Work out the finished part from the listing and answer in its coordinate system (mm). Give positions to 0.01 mm unless a question says otherwise; leave off trailing zeros. Write each loop counter-clockwise with the first axis right and the second up, starting at its lowest first coordinate (ties: lowest second). Pieces come first, ordered by that corner, then holes.
1) Find section A-A (z = 2.5). Determine the outline of the cut face in (x, y), plus the area to 3 significant figures.
2) Determine the mould class of faces 1 (the face through (2.49, -0.13, 3.49)), 2 (the face through (2.5, 0, 4)), 3 (the face through (-38, 0, -3)) for opening direction Z: pulls with the +Z half, pulls with the -Z half, needs draft (parallel to the pull), parting line crosses it, or undercut.
3) Given pin 1 Ø4 at (x, z) = (-20.5, -3) entering from +Y; pin 2 Ø3 at (y, z) = (0, -7.5) entering from -X; pin 3 Ø3 at (x, y) = (-32, 0.5) entering from +Z, each flat-ended and moving along its own axis, determine where each tip first touches the part or whether it passes through.
4) Find section C-C (x = -18.5). Determine the outline of the cut face in (y, z), plus the area to 3 significant figures.
5) Find section B-B (y = -0.4). Determine the outline of the cut face in (x, z), plus the area to 3 significant figures.
6) Straight lines are drawn through the part: probe 1 along Z at (x, y) = (2.7, 0); probe 2 along Y at (x, z) = (2.45, -7.5); probe 3 along X at (y, z) = (-1.15, -1.75). For each, find the intervals that lie inside material, in ascending order.
7) Find section D-D (z = -0.5). Determine the outline of the cut face in (x, y).
```python
from build123d import *

# Parameters (mm, degrees)
SKETCH_1_W          = 4
SKETCH_1_H          = 6
SKETCH_1_R          = 1
EXTRUDE_1_DEPTH     = 1
SKETCH_2_W          = 3
SKETCH_2_H          = 6
SKETCH_2_R          = 1
SKETCH_2_W_2        = 3.5
EXTRUDE_2_DEPTH     = 1
FILLET_1_R          = 1
SKETCH_3_W          = 8.324991738
SKETCH_3_H          = 7.604036572
CUT_EXTRUDE_1_DEPTH = 10
EXTRUDE_3_DEPTH     = 40


with BuildPart() as part:
    # 草图1 → 凸台-拉伸1 (new body)
    with BuildSketch(Plane.XY):
        Rectangle(SKETCH_1_W, SKETCH_1_H)
        Circle(SKETCH_1_R, mode=Mode.SUBTRACT)
    extrude(amount=EXTRUDE_1_DEPTH)

    # 草图2 → 凸台-拉伸2 (add)
    # profile 1 of 2: a face of its own
    with BuildSketch(Plane(origin=(2, 0, 0), x_dir=(0, 0, -1), z_dir=(1, 0, 0))):
        with Locations((-2.5, 0)):
            Rectangle(SKETCH_2_W, SKETCH_2_H)
        with Locations(Location((-2.5, 0, 0), (0, 0, 90))):
            Circle(SKETCH_2_R, mode=Mode.SUBTRACT)
    # profile 2 of 2: a face of its own
    with BuildSketch(Plane(origin=(2, 0, 0), x_dir=(0, 0, -1), z_dir=(1, 0, 0))):
        with Locations((0.75, 0)):
            Rectangle(SKETCH_2_W_2, SKETCH_2_H)
    extrude(amount=EXTRUDE_2_DEPTH)

    # 圆角1
    fillet_1_edges = [part.edges().sort_by_distance(p)[0] for p in [
        (-2, -3, 0.5),
        (-2, 3, 0.5),
    ]]
    fillet(fillet_1_edges, radius=FILLET_1_R)

    # 镜向1: part across plane


with BuildPart() as part_1:
    add(part.part)
    add(part.part.mirror(Plane(origin=(3, 0, -2.5), x_dir=(1, 0, 0), z_dir=(0, 0, 1))))

    # 草图3 → 切除-拉伸1 (cut)
    with BuildSketch(Plane.ZY.offset(-2)):
        with Locations((-2.5, 0)):
            Rectangle(SKETCH_3_W, SKETCH_3_H)
    extrude(amount=CUT_EXTRUDE_1_DEPTH, mode=Mode.SUBTRACT)

    # 草图4 → 凸台-拉伸3 (add)
    with BuildSketch(Plane.ZY.offset(-2)):
        with BuildLine():
            ThreePointArc((-1.5, 0), (-1.792893219, 0.707106781), (-2.5, 1))
            Line((-2.5, 1), (-2.5, 0))
            Line((-2.5, 0), (-1.5, 0))
        make_face()
        with BuildLine():
            Line((-2.5, 0), (-2.5, 1))
            ThreePointArc((-2.5, 1), (-3.207106781, 0.707106781), (-3.5, 0))
            Line((-3.5, 0), (-2.5, 0))
        make_face()
        with BuildLine():
            Line((-1.5, 0), (-2.5, 0))
            Line((-2.5, 0), (-2.5, -1))
            ThreePointArc((-2.5, -1), (-1.792893219, -0.707106781), (-1.5, 0))
        make_face()
        with BuildLine():
            Line((-2.5, -1), (-2.5, 0))
            Line((-2.5, 0), (-3.5, 0))
            ThreePointArc((-3.5, 0), (-3.207106781, -0.707106781), (-2.5, -1))
        make_face()
    extrude(amount=EXTRUDE_3_DEPTH)


solid = part_1.part
```
Results:
1. outline: (2, -3) - (3, -3) - (3, -1) - (2, -1) - close; (2, 1) - (3, 1) - (3, 3) - (2, 3) - close
1. area: 4.00 mm2
2. face 1: undercut
2. face 2: pulls with the +Z half
2. face 3: needs draft
3. pin 1: stops at y = 1
3. pin 2: stops at x = 2
3. pin 3: stops at z = -1.5
4. outline: circle Ø2 at (0, -2.5)
4. area: 3.14 mm2
5. outline: (-38, -3.42) - (2, -3.42) - (2, -6.58) - (3, -6.58) - (3, 1.58) - (2, 1.58) - (2, -1.58) - (-38, -1.58) - close; (2, -9) - (3, -9) - (3, -8.42) - (2, -8.42) - close; (2, 3.42) - (3, 3.42) - (3, 4) - (2, 4) - close
5. area: 82.7 mm2
6. probe 1: z = -9 to -8.5, -6.5 to 1.5, 3.5 to 4
6. probe 2: y = -3 to -1, 1 to 3
6. probe 3: x = 2 to 3
7. outline: (2, -3) - (3, -3) - (3, 3) - (2, 3) - close
